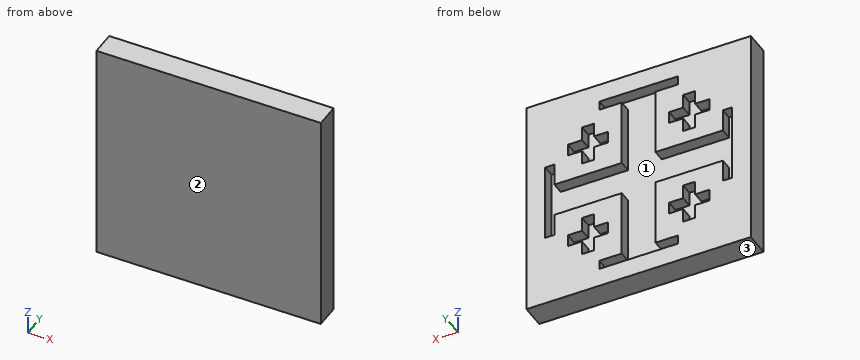
from build123d import *

# Parameters (mm, degrees)
SKETCH1_W           = 47.625
SKETCH1_H           = 47.625
BOSS_EXTRUDE1_DEPTH = 5.15
CUT_EXTRUDE1_DEPTH  = 2.54


with BuildPart() as part:
    # Sketch1 → Boss-Extrude1 (new body)
    with BuildSketch(Plane(origin=(0, 0, 0), x_dir=(1, 0, 0), z_dir=(0, 1, 0))):
        with Locations((23.8125, 23.8125)):
            Rectangle(SKETCH1_W, SKETCH1_H)
    extrude(amount=BOSS_EXTRUDE1_DEPTH)

    # Sketch2 → Cut-Extrude1 (cut)
    with BuildSketch(Plane(origin=(0, 5.15, 0), x_dir=(1, 0, 0), z_dir=(0, 1, 0))):
        Polygon((20.234147834, 27.390852166), (5.928370013, 27.390852166), (5.928370013, 32.150779252), (3.990438648, 32.150779252), (3.990438648, 15.474220748), (5.928370013, 15.474220748), (5.928370013, 20.234147834), (20.234147834, 20.234147834), (20.234147834, 5.928370013), (15.474220748, 5.928370013), (15.474220748, 3.990438648), (32.150779252, 3.990438648), (32.150779252, 5.928370013), (27.390852166, 5.928370013), (27.390852166, 20.234147834), (41.696629987, 20.234147834), (41.696629987, 15.474220748), (43.634561352, 15.474220748), (43.634561352, 32.150779252), (41.696629987, 32.150779252), (41.696629987, 27.390852166), (27.390852166, 27.390852166), (27.390852166, 41.696629987), (32.150779252, 41.696629987), (32.150779252, 43.634561352), (15.474220748, 43.634561352), (15.474220748, 41.696629987), (20.234147834, 41.696629987), align=None)
        Polygon((17.356946081, 35.819869232), (17.356946081, 33.26761292), (14.35738708, 33.26761292), (14.35738708, 30.268053919), (11.805130768, 30.268053919), (11.805130768, 33.26761292), (8.805571767, 33.26761292), (8.805571767, 35.819869232), (11.805130768, 35.819869232), (11.805130768, 38.819428233), (14.35738708, 38.819428233), (14.35738708, 35.819869232), align=None)
        Polygon((35.819869232, 30.268053919), (33.26761292, 30.268053919), (33.26761292, 33.26761292), (30.268053919, 33.26761292), (30.268053919, 35.819869232), (33.26761292, 35.819869232), (33.26761292, 38.819428233), (35.819869232, 38.819428233), (35.819869232, 35.819869232), (38.819428233, 35.819869232), (38.819428233, 33.26761292), (35.819869232, 33.26761292), align=None)
        Polygon((30.268053919, 11.805130768), (30.268053919, 14.35738708), (33.26761292, 14.35738708), (33.26761292, 17.356946081), (35.819869232, 17.356946081), (35.819869232, 14.35738708), (38.819428233, 14.35738708), (38.819428233, 11.805130768), (35.819869232, 11.805130768), (35.819869232, 8.805571767), (33.26761292, 8.805571767), (33.26761292, 11.805130768), align=None)
        Polygon((11.805130768, 17.356946081), (14.35738708, 17.356946081), (14.35738708, 14.35738708), (17.356946081, 14.35738708), (17.356946081, 11.805130768), (14.35738708, 11.805130768), (14.35738708, 8.805571767), (11.805130768, 8.805571767), (11.805130768, 11.805130768), (8.805571767, 11.805130768), (8.805571767, 14.35738708), (11.805130768, 14.35738708), align=None)
    extrude(amount=-CUT_EXTRUDE1_DEPTH, mode=Mode.SUBTRACT)


solid = part.part
Could you check a few things on this model? Use its own coordinates, in mm. Face numbers are marked on the shaded views. Coordinates: 2 decimals unless noted, no trailing zeros. Write each loop counter-clockwise with the first axis right and the second up, starting at its lowest first coordinate (ties: lowest second). Pieces come first, ordered by that corner, then holes. Notation, with made-up numbers: (32.25, 50.25) - (90.25, 50.25) arc R29 cw to (90.25, 76.25) - close; hole circle Ø1 at (28.25, 35). An arc over 180 degrees is marked (long way). Write item = value, one per line.
1) Suppose I cut it at B-B on z = -31.5. Please give me the cut outline in (x, y) (3 decimals).
Result set:
outline = (0, 0) - (47.625, 0) - (47.625, 5.15) - (43.635, 5.15) - (43.635, 2.61) - (41.697, 2.61) - (41.697, 5.15) - (35.82, 5.15) - (35.82, 2.61) - (33.268, 2.61) - (33.268, 5.15) - (27.391, 5.15) - (27.391, 2.61) - (20.234, 2.61) - (20.234, 5.15) - (14.357, 5.15) - (14.357, 2.61) - (11.805, 2.61) - (11.805, 5.15) - (5.928, 5.15) - (5.928, 2.61) - (3.99, 2.61) - (3.99, 5.15) - (0, 5.15) - close
2) Please list where these lines run through material, in increasing order: line 1 (X direction, y = 3.15, z = -10.5) (3 decimals); line 2 (Z direction, x = 37, y = 4.1) (3 decimals); line 3 (X direction, y = 4.2, z = -16) (3 decimals). Write a range as [from, to].
Result set:
line_1 = [0, 11.805], [14.357, 20.234], [27.391, 33.268], [35.82, 47.625]
line_2 = [-47.625, -35.82], [-33.268, -27.391], [-20.234, -14.357], [-11.805, 0]
line_3 = [0, 3.99], [5.928, 11.805], [14.357, 20.234], [27.391, 33.268], [35.82, 41.697], [43.635, 47.625]
3) We'd pull the mould along Z, two halves only. Please class the marked faces 1, 2 and 3: +Z half, -Z half, draft (parallel to the pull), parting line (faces both ways), or undercut.
Result set:
face_1 = undercut
face_2 = draft
face_3 = -Z half
4) Suppose I cut it at C-C on y = 4.6. State how many separate pieces and enclosed holes the cut face has, plus the area to 3 significant figures.
Result set:
separate_pieces = 1
enclosed_holes = 5
area = 1,530 mm2
5) Suppose I cut it at A-A on x = 34. Please give me the cut outline in (y, z) (3 decimals).
Result set:
outline = (0, -47.625) - (5.15, -47.625) - (5.15, -38.819) - (2.61, -38.819) - (2.61, -30.268) - (5.15, -30.268) - (5.15, -27.391) - (2.61, -27.391) - (2.61, -20.234) - (5.15, -20.234) - (5.15, -17.357) - (2.61, -17.357) - (2.61, -8.806) - (5.15, -8.806) - (5.15, 0) - (0, 0) - close
6) Suppose I cut it at D-D on z = -6.5. Please give me the cut outline in (x, y) (3 decimals).
Result set:
outline = (0, 0) - (47.625, 0) - (47.625, 5.15) - (27.391, 5.15) - (27.391, 2.61) - (20.234, 2.61) - (20.234, 5.15) - (0, 5.15) - close
